Design review of the part built by this model. Coordinates are the model's own, in mm. A direction names the side the tool comes from. Round coordinates to 2 decimals unless told otherwise and drop trailing zeros. Order: outer loops, then holes, each group sorted by start corner. A loop starts at its lowest first (then second) coordinate and runs counter-clockwise, first axis right, second up.
from build123d import *

# Parameters (mm, degrees)
SKETCH_1_R          = 2.95
EXTRUDE_1_DEPTH     = 2.9
SKETCH_2_R          = 1.5
EXTRUDE_2_DEPTH     = 14
SKETCH_3_R          = 1.25
EXTRUDE_3_DEPTH     = 5
CUT_EXTRUDE_1_DEPTH = 2
FILLET_1_R          = 0.2


with BuildPart() as part:
    # 草图1 → 凸台-拉伸1 (new body)
    with BuildSketch(Plane(origin=(0, 0, 0), x_dir=(1, 0, 0), z_dir=(0, 1, 0))):
        with Locations(Location((0, 0, 0), (0, 0, 270))):
            Circle(SKETCH_1_R)
    extrude(amount=EXTRUDE_1_DEPTH)

    # 草图2 → 凸台-拉伸2 (add)
    with BuildSketch(Plane(origin=(0, 2.9, 0), x_dir=(1, 0, 0), z_dir=(0, 1, 0))):
        with Locations(Location((0, 0, 0), (0, 0, 270))):
            Circle(SKETCH_2_R)
    extrude(amount=EXTRUDE_2_DEPTH)

    # 草图3 → 凸台-拉伸3 (add)
    with BuildSketch(Plane(origin=(0, 16.9, 0), x_dir=(1, 0, 0), z_dir=(0, 1, 0))):
        with Locations(Location((0, 0, 0), (0, 0, 270))):
            Circle(SKETCH_3_R)
    extrude(amount=EXTRUDE_3_DEPTH)

    # 草图4 → 切除-拉伸1 (cut)
    with BuildSketch(Plane.XZ):
        Polygon((2.247285488, -0.53201623), (1.584382314, 1.680198207), (-0.662903174, 2.212214437), (-2.247285488, 0.53201623), (-1.584382314, -1.680198207), (0.662903174, -2.212214437), align=None)
    extrude(amount=-CUT_EXTRUDE_1_DEPTH, mode=Mode.SUBTRACT)

    # 圆角1
    fillet_1_edges = [part.edges().sort_by_distance(p)[0] for p in [
        (0, 21.9, -1.25),
        (0, 0, -2.95),
        (0, 2.9, -2.95),
    ]]
    fillet(fillet_1_edges, radius=FILLET_1_R)


solid = part.part
1) Take a section at C-C on x = 0. Give the boundary of the cut face in (y, z), plus the area to 3 significant figures.
Results:
outline: (0, -2.75) arc R0.2 ccw to (0.2, -2.95) - (2.7, -2.95) arc R0.2 ccw to (2.9, -2.75) - (2.9, -1.5) - (16.9, -1.5) - (16.9, -1.25) - (21.7, -1.25) arc R0.2 ccw to (21.9, -1.05) - (21.9, 1.05) arc R0.2 ccw to (21.7, 1.25) - (16.9, 1.25) - (16.9, 1.5) - (2.9, 1.5) - (2.9, 2.75) arc R0.2 ccw to (2.7, 2.95) - (0.2, 2.95) arc R0.2 ccw to (0, 2.75) - (0, 2.06) - (2, 2.06) - (2, -2.06) - (0, -2.06) - close
area: 63.3 mm2
2) Take a section at B-B on y = 9.5. Give the boundary of the cut face in (x, z).
Results:
outline: circle Ø3 at (0, 0)
3) To check wall thickness, follow line 1 along Y through (x, z) = (2.65, -0.6); line 2 along Y through (x, z) = (1.3, -1.25); line 3 along X through (y, z) = (1.75, 0.2). State the ranges of each line that lie inside material, in increasing order.
Results:
line 1: y = 0 to 2.9
line 2: y = 2 to 2.9
line 3: x = -2.94 to -2.15, 2.03 to 2.94
4) For faces 1 (the face through (-2.88, 1.43, -0.64)), 2 (the face through (-1.92, 0.99, -0.56)), 3 (the face through (0.45, 9.8, 1.43)), list the 3-axis set-ups (+Z, -Z, +X, -X, +Y, -Y) from which the entire face can be reached by the end or side of a thin tool; tool diameter is ignored.
Results:
face 1: +Y, -Y
face 2: -Y
face 3: +Y
5) The part is to be moulded in two halves that separate along Z. For faces 4 (the face through (-1.2, 2.9, 1.2)), 5 (the face through (1.444, 0.986, -1.384)), 6 (the face through (1.92, 0.99, 0.56)), 7 (the face through (-1.22, 19.27, -0.27)), say which applies: released by +Z, released by -Z, zero draft, split by the parting line, or undercut.
Results:
face 4: zero draft
face 5: undercut
face 6: undercut
face 7: split by the parting line
6) Clearance check with flat-ended pins moving along their axes: P1, Ø1.5, axis at y = 3.5, z = 0.5, coming from the -X side; P2, Ø1.5, axis at y = 11, z = -2, coming from the +X side; P3, Ø3.5, axis at x = 0, z = 0, coming from the -Y side. State where each tip first meets the part, or that it passes through.
Results:
P1: stops at x = -2.92
P2: stops at x = 0.83
P3: stops at y = 2
7) Take a section at A-A on z = 0. Give the boundary of the cut face in (x, y), plus the area to 3 significant figures.
Results:
outline: (-2.95, 0.2) arc R0.2 ccw to (-2.75, 0) - (-2.09, 0) - (-2.09, 2) - (2.09, 2) - (2.09, 0) - (2.75, 0) arc R0.2 ccw to (2.95, 0.2) - (2.95, 2.7) arc R0.2 ccw to (2.75, 2.9) - (1.5, 2.9) - (1.5, 16.9) - (1.25, 16.9) - (1.25, 21.7) arc R0.2 ccw to (1.05, 21.9) - (-1.05, 21.9) arc R0.2 ccw to (-1.25, 21.7) - (-1.25, 16.9) - (-1.5, 16.9) - (-1.5, 2.9) - (-2.75, 2.9) arc R0.2 ccw to (-2.95, 2.7) - close
area: 63.2 mm2
